```python
from build123d import *

# Parameters (mm, degrees)
F0_R     = 3.895446
F1_DEPTH = 152.4
F5_DEPTH = 4.572


with BuildPart() as f1:
    # F0 (on Front) → F1 (new body)
    with BuildSketch(Plane.XZ):
        with Locations((-66.586629, 45.847487)):
            Circle(F0_R)
    extrude(amount=F1_DEPTH)

    # F2 (on face) → F5 (join)
    with BuildSketch(Plane.XZ.offset(152.4)):
        Polygon((-70.592547, 38.909033), (-62.58071, 38.909033), (-58.574792, 45.847487), (-62.58071, 52.78594), (-70.592547, 52.78594), (-74.598465, 45.847487), align=None)
    extrude(amount=F5_DEPTH)


with BuildPart() as f3_1:
    # F3: copy of F1
    add(f1.part.moved(Location((-51.054, 57.15, -154.94))))


solid = f1.part
```
Work out the finished part from the listing and answer in its coordinate system (mm). A direction names the side the tool comes from. Coordinates: 2 decimals unless noted, no trailing zeros. Loops run counter-clockwise (first coordinate to the right, second up) from the corner with the lowest first, then second, coordinate; pieces in that order, holes last.
1) Consider probe 1 along Y at (x, z) = (-64.5, 40.25); probe 2 along Z at (x, y) = (-67, -22); probe 3 along X at (y, z) = (-32, 42.5). Determine where each line is inside the solid, lowest interval first.
Results:
probe 1: y = -156.97 to -152.4
probe 2: z = 41.97 to 49.72
probe 3: x = -68.58 to -64.59
2) Section B-B (z = 43.75) is taken. Give the vertices of the cut face in (x, y), plus the area to 3 significant figures.
Results:
outline: (-73.39, -156.97) - (-59.79, -156.97) - (-59.79, -152.4) - (-63.3, -152.4) - (-63.3, 0) - (-69.87, 0) - (-69.87, -152.4) - (-73.39, -152.4) - close
area: 1,060 mm2
3) Section C-C (y = -31.5) is taken. Give the vertices of the cut face in (x, z).
Results:
outline: circle Ø7.79 at (-66.59, 45.85)
4) Flat-ended cylindrical pins translate along their axes: pin 1 (6 mm diameter, centred on x = -62.5, z = 41, fed in from +Y); pin 2 (1.5 mm diameter, centred on y = -138, z = 42, fed in from -X); pin 3 (1 mm diameter, centred on x = -61, y = -43.5, fed in from +Z); pin 4 (2 mm diameter, centred on x = -70, y = -66, fed in from +Z). Find the tip coordinate at first contact, or state that the pin passes through.
Results:
pin 1: stops at y = 0
pin 2: stops at x = -68.95
pin 3: passes through
pin 4: stops at z = 48.91
5) Section D-D (x = -73.25) is taken. Give the vertices of the cut face in (y, z).
Results:
outline: (-156.97, 43.51) - (-152.4, 43.51) - (-152.4, 48.18) - (-156.97, 48.18) - close
6) For faces 1 (the flat face through (-72.567, -154.654, 49.365)), 2 (the cylindrical face through (-62.87, -75.13, 47.02)), determine the directions among +Z, -Z, +X, -X, +Y, -Y from which every point of the face is accessible in a straight line to the end or side of a thin tool.
Results:
face 1: +Z, -X, +Y, -Y
face 2: +Y
7) Section A-A (x = -64.5) is taken. Give the vertices of the cut face in (y, z).
Results:
outline: (-156.97, 38.91) - (-152.4, 38.91) - (-152.4, 42.56) - (0, 42.56) - (0, 49.14) - (-152.4, 49.14) - (-152.4, 52.79) - (-156.97, 52.79) - close
